Here's the drawing with two shaded views (mm, measured from the low corner). I have some questions. Give positions to 0.01 mm unless a question says otherwise; leave off trailing zeros. Write each loop counter-clockwise with the first axis right and the second up, starting at its lowest first coordinate (ties: lowest second). Pieces come first, ordered by that corner, then holes.
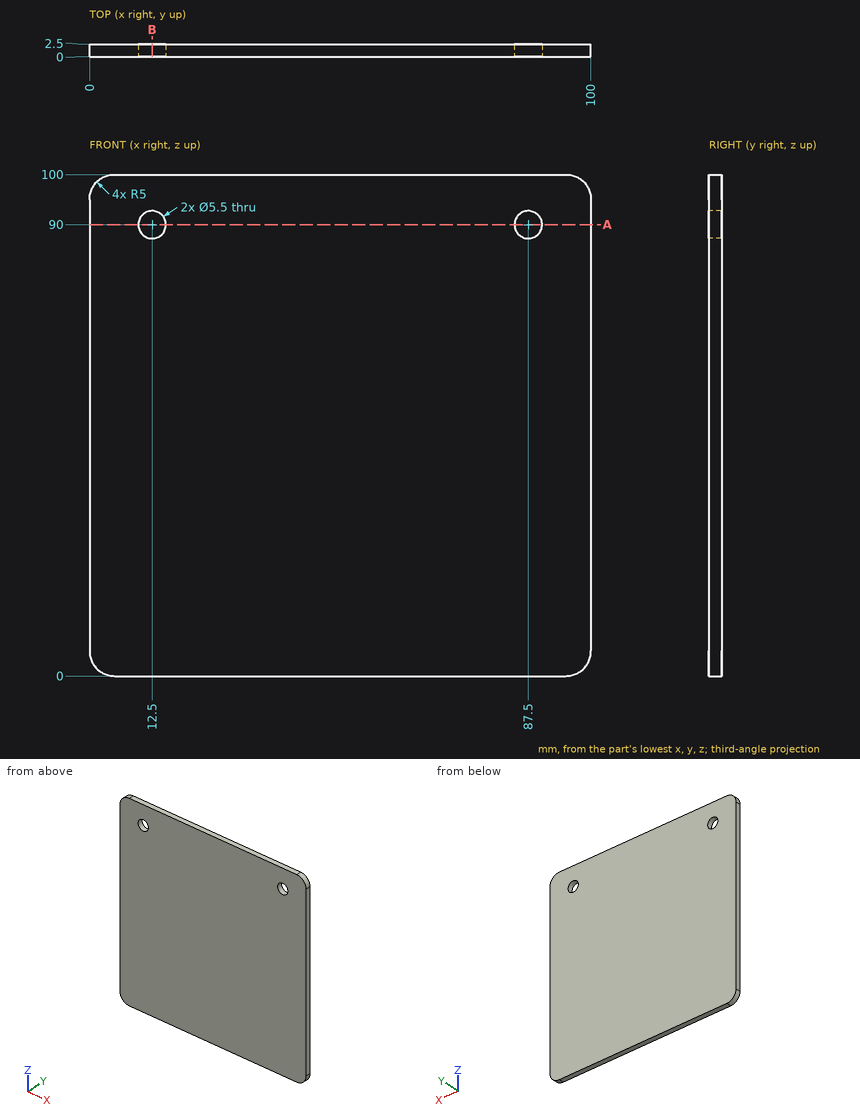
1) Suppose I cut it at A-A on z = 90. Write out the boundary of the cut face in (x, y), plus the area to 4 significant figures.
Values follow:
outline: (0, 0) - (9.75, 0) - (9.75, 2.5) - (0, 2.5) - close; (15.25, 0) - (84.75, 0) - (84.75, 2.5) - (15.25, 2.5) - close; (90.25, 0) - (100, 0) - (100, 2.5) - (90.25, 2.5) - close
area: 222.5 mm2
2) Please list where these lines run through material, in increasing order: L1, parallel to X at y = 1.95, z = 90; L2, parallel to Z at x = 12.5, y = 1.4.
Values follow:
L1: x = 0 to 9.75, 15.25 to 84.75, 90.25 to 100
L2: z = 0 to 87.25, 92.75 to 100
3) Suppose I cut it at B-B on x = 12.5. Write out the boundary of the cut face in (y, z), plus the area to 3 significant figures.
Values follow:
outline: (0, 0) - (2.5, 0) - (2.5, 87.25) - (0, 87.25) - close; (0, 92.75) - (2.5, 92.75) - (2.5, 100) - (0, 100) - close
area: 236 mm2
